Job drawing, mm, ordinate dimensions from the low corner. One solid piece. A direction names the side the tool comes from. Give positions to 0.01 mm unless a question says otherwise; leave off trailing zeros. Order: outer loops, then holes, each group sorted by start corner. A loop starts at its lowest first (then second) coordinate and runs counter-clockwise, first axis right, second up.
1. Slice it at A-A on y = 100. List the corners of the cut face in (x, z).
2. Which spindle directions (+Z, -Z, +X, -X, +Y, -Y) get a long thin tool onto all of the face, cutting with end or side? Do the marked faces 4 and 5. Say none if no direction does.
3. Mould opens along X. For the marked faces 1, 2 and 3 say: +X half, -X half, draft (parallel to the pull), parting line (faces both ways), or undercut.
4. Slice it at C-C on z = 6.25. List the corners of the cut face in (x, y).
5. Slice it at D-D on x = 6. List the corners of the cut face in (y, z).
6. Drop a flat-ended pin along its axis: pin 1 Ø1.5 at (x, y) = (35, 93.5) entering from +Z. Give the stop position or say it passes through.
7. Slice it at B-B on x = 47. List the corners of the cut face in (y, z), and give its area (3 significant figures).
8. Probe line 1 (Y direction, x = 53, z = 6.25); line 2 (X direction, y = 104, z = 6.5); line 3 (Z direction, x = 19, y = 65.5). List the from-to ranges inside material, lowest first.
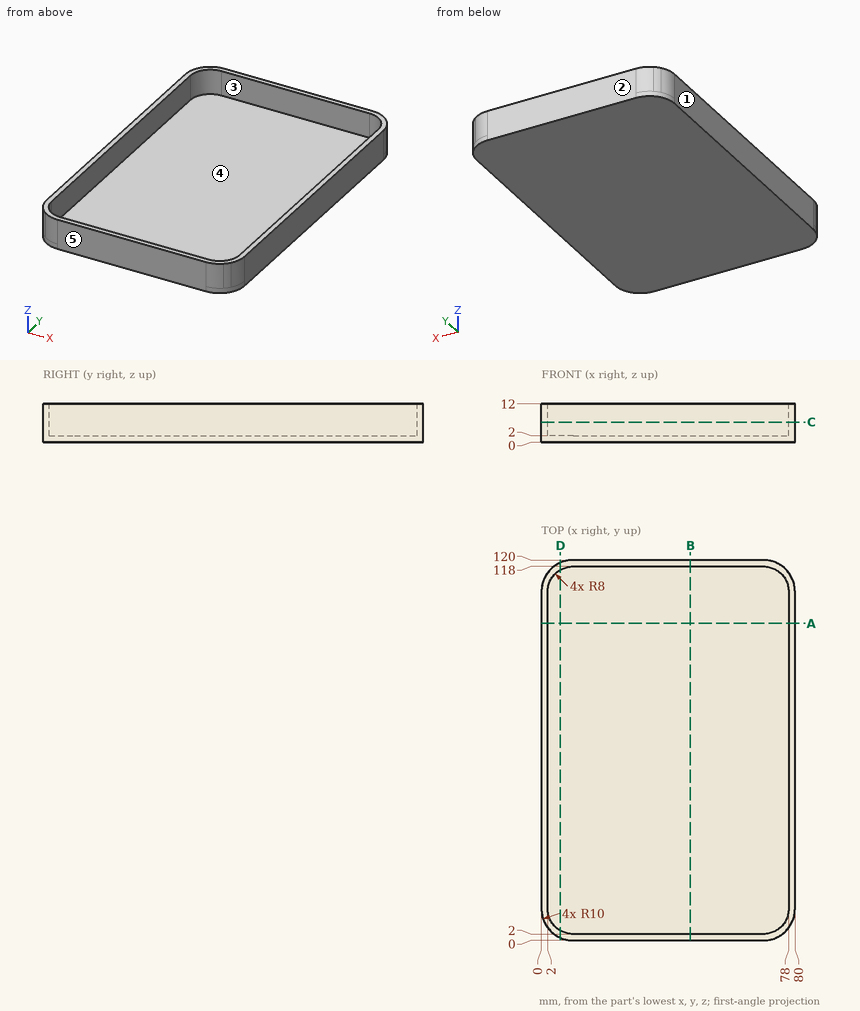
Data:
1. outline: (0, 0) - (80, 0) - (80, 12) - (78, 12) - (78, 2) - (2, 2) - (2, 12) - (0, 12) - close
2. face 4: +Z
2. face 5: +Z, -Z, +X, -X, -Y
3. face 1: -X half
3. face 2: draft
3. face 3: undercut
4. outline: (0, 10) arc R10 ccw to (10, 0) - (70, 0) arc R10 ccw to (80, 10) - (80, 110) arc R10 ccw to (70, 120) - (10, 120) arc R10 ccw to (0, 110) - close; hole (2, 10) arc R8 ccw to (10, 2) - (70, 2) arc R8 ccw to (78, 10) - (78, 110) arc R8 ccw to (70, 118) - (10, 118) arc R8 ccw to (2, 110) - close
5. outline: (0.83, 0) - (119.17, 0) - (119.17, 12) - (116.93, 12) - (116.93, 2) - (3.07, 2) - (3.07, 12) - (0.83, 12) - close
6. pin 1: stops at z = 2
7. outline: (0, 0) - (120, 0) - (120, 12) - (118, 12) - (118, 2) - (2, 2) - (2, 12) - (0, 12) - close
7. area: 280 mm2
8. line 1: y = 0 to 2, 118 to 120
8. line 2: x = 0 to 2, 78 to 80
8. line 3: z = 0 to 2
